Check sheet for the modelled part. Datum: model origin and axes. Units: mm. A direction names the side the tool comes from. Round coordinates to 2 decimals unless told otherwise and drop trailing zeros. Loops run counter-clockwise (first coordinate to the right, second up) from the corner with the lowest first, then second, coordinate; pieces in that order, holes last. Notation, with made-up numbers: (2, 50.25) - (49, 50.25) arc R15 cw to (49, 69.25) - close; hole circle Ø4 at (-11, -31). An arc over 180 degrees is marked (long way). Put each result on its own line as item: value.
```python
from build123d import *

# Parameters (mm, degrees)
SKETCH_1_W           = 1100
SKETCH_1_H           = 800
EXTRUDE_1_DEPTH      = 6
SKETCH_3_W           = 1100
SKETCH_3_H           = 800
SKETCH_3_W_2         = 1088
SKETCH_3_H_2         = 788
EXTRUDE_2_DEPTH      = 1200
SKETCH_4_W           = 900
SKETCH_4_H           = 800
EXTRUDE_3_DEPTH      = 4
SKETCH_5_W           = 50
SKETCH_5_H           = 50
EXTRUDE_4_DEPTH      = 950
EXTRUDE_5_DEPTH      = 19
EXTRUDE_5_DEPTH_BACK = 800
SKETCH_6_R           = 44.5
SKETCH_6_R_2         = 41
SKETCH_7_R           = 28.5
SKETCH_7_R_2         = 25
EXTRUDE_6_DEPTH      = 50
EXTRUDE_7_DEPTH      = 50
EXTRUDE_7_DEPTH_BACK = 50
SKETCH_8_R           = 16.75
SKETCH_8_R_2         = 13.55
SKETCH_9_R           = 21.15
SKETCH_9_R_2         = 17.95
EXTRUDE_8_DEPTH      = 49
SKETCH_10_R          = 16.75
SKETCH_10_R_2        = 13.55
EXTRUDE_9_DEPTH      = 30
SKETCH_13_W          = 1100
SKETCH_13_H          = 4
EXTRUDE_12_DEPTH     = 160
SKETCH_14_R          = 16.75
SKETCH_14_R_2        = 13.55
EXTRUDE_13_DEPTH     = 30


with BuildPart() as part:
    # Эскиз1 → Бобышка-Вытянуть1 (new body)
    with BuildSketch(Plane(origin=(0, 0, 0), x_dir=(1, 0, 0), z_dir=(0, 1, 0))):
        with Locations((550, 400)):
            Rectangle(SKETCH_1_W, SKETCH_1_H)
    extrude(amount=EXTRUDE_1_DEPTH)

    # Эскиз3 → Бобышка-Вытянуть2 (add)
    with BuildSketch(Plane(origin=(0, 6, 0), x_dir=(1, 0, 0), z_dir=(0, 1, 0))):
        with Locations((550, 400)):
            Rectangle(SKETCH_3_W, SKETCH_3_H)
        with Locations((550, 400)):
            Rectangle(SKETCH_3_W_2, SKETCH_3_H_2, mode=Mode.SUBTRACT)
    extrude(amount=EXTRUDE_2_DEPTH)

    # Эскиз4 → Бобышка-Вытянуть3 (add)
    with BuildSketch(Plane(origin=(0, 1206, 0), x_dir=(1, 0, 0), z_dir=(0, 1, 0))):
        with Locations((650, 400)):
            Rectangle(SKETCH_4_W, SKETCH_4_H)
    extrude(amount=EXTRUDE_3_DEPTH)

    # Эскиз5 → Бобышка-Вытянуть4 (add)
    with BuildSketch(Plane.XZ):
        with Locations((1075, -25)):
            Rectangle(SKETCH_5_W, SKETCH_5_H)
        with Locations((25, -25)):
            Rectangle(SKETCH_5_W, SKETCH_5_H)
        with Locations((1075, -775)):
            Rectangle(SKETCH_5_W, SKETCH_5_H)
        with Locations((25, -775)):
            Rectangle(SKETCH_5_W, SKETCH_5_H)
    extrude(amount=EXTRUDE_4_DEPTH)

    # Эскиз6 → Бобышка-Вытянуть5 (add, two sides: drawn at the far end of the back side and taken through both)
    with BuildSketch(Plane(origin=(0, 1210, 0), x_dir=(1, 0, 0), z_dir=(0, 1, 0)).offset(-EXTRUDE_5_DEPTH_BACK)):
        with Locations(Location((1000, 100, 0), (0, 0, 270))):
            Circle(SKETCH_6_R)
        with Locations(Location((1000, 100, 0), (0, 0, 270))):
            Circle(SKETCH_6_R_2, mode=Mode.SUBTRACT)
    extrude(amount=EXTRUDE_5_DEPTH + EXTRUDE_5_DEPTH_BACK)

    # Эскиз7 → Бобышка-Вытянуть6 (add)
    with BuildSketch(Plane.ZY):
        with Locations(Location((-250, 1160, 0), (0, 0, 180))):
            Circle(SKETCH_7_R)
        with Locations((-250, 1160)):
            Circle(SKETCH_7_R_2, mode=Mode.SUBTRACT)
    extrude(amount=EXTRUDE_6_DEPTH)

    # Эскиз8 → Бобышка-Вытянуть7 (add, two sides: drawn at the far end of the back side and taken through both)
    with BuildSketch(Plane.XZ.offset(-EXTRUDE_7_DEPTH_BACK)):
        with Locations(Location((171.2, -100, 0), (0, 0, 270))):
            Circle(SKETCH_8_R)
        with Locations(Location((171.2, -100, 0), (0, 0, 270))):
            Circle(SKETCH_8_R_2, mode=Mode.SUBTRACT)
    extrude(amount=EXTRUDE_7_DEPTH + EXTRUDE_7_DEPTH_BACK)

    # Эскиз9 → Бобышка-Вытянуть8 (add)
    with BuildSketch(Plane.XZ):
        with Locations(Location((300, -250, 0), (0, 0, 270))):
            Circle(SKETCH_9_R)
        with Locations(Location((300, -250, 0), (0, 0, 270))):
            Circle(SKETCH_9_R_2, mode=Mode.SUBTRACT)
    extrude(amount=EXTRUDE_8_DEPTH)

    # Эскиз10 → Бобышка-Вытянуть9 (add)
    with BuildSketch(Plane.XY):
        with Locations(Location((500, 1150, 0), (0, 0, 180))):
            Circle(SKETCH_10_R)
        with Locations((500, 1150)):
            Circle(SKETCH_10_R_2, mode=Mode.SUBTRACT)
    extrude(amount=EXTRUDE_9_DEPTH)

    # Эскиз13 → Бобышка-Вытянуть12 (add)
    with BuildSketch(Plane.XY):
        with Locations((550, -752)):
            Rectangle(SKETCH_13_W, SKETCH_13_H)
    extrude(amount=EXTRUDE_12_DEPTH)

    # Эскиз14 → Бобышка-Вытянуть13 (add)
    with BuildSketch(Plane.XY):
        with Locations(Location((550, 50, 0), (0, 0, 180))):
            Circle(SKETCH_14_R)
        with Locations((550, 50)):
            Circle(SKETCH_14_R_2, mode=Mode.SUBTRACT)
    extrude(amount=EXTRUDE_13_DEPTH)


solid = part.part
```
Item 1: Section check A-A on y = 583. Enter the section's corners in (x, z), then the cut area to 3 significant figures.
Filled sheet:
outline: (0, -800) - (1100, -800) - (1100, 0) - (0, 0) - close; circle Ø89 at (1000, -100); hole (6, -794) - (1094, -794) - (1094, -6) - (6, -6) - close; hole circle Ø82 at (1000, -100)
area: 23,600 mm²
Item 2: Section check C-C on z = -502.5. Enter the section's corners in (x, y).
Filled sheet:
outline: (0, 0) - (1100, 0) - (1100, 1210) - (200, 1210) - (200, 1206) - (1094, 1206) - (1094, 6) - (6, 6) - (6, 1206) - (0, 1206) - close
Item 3: Thickness scan on line 1 (Z direction, x = 171.2, y = 16); line 2 (Y direction, x = 550, z = 7.75); line 3 (Y direction, x = 687.5, z = -36). Record the ranges inside material, lowest first. Write a range as from..to.
Filled sheet:
line 1: -800..-794, -116.75..-113.55, -86.45..-83.25, -6..0
line 2: -754..-750, 33.25..36.45, 63.55..66.75
line 3: 0..6, 1206..1210
Item 4: Go/stop test with flat-tipped pins: pin 1 (10 mm diameter, centred on y = 33, z = -613.5, fed in from -X); pin 2 (8 mm diameter, centred on x = 521, z = -405.5, fed in from -Y). Record where each tip stops, or that it passes through.
Filled sheet:
pin 1: x = 0
pin 2: y = 0
Item 5: Tool access check on faces 1 (the cylindrical face through (956.56, 1219.37, -109.65)), 2 (the flat face through (25, -468, -50)), 3 (the flat face through (542, 6, -406)). Record the directions out of +Z, -Z, +X, -X, +Y, -Y that give a thin tool (end or side, any length) a straight path to the whole face; none if there is none.
Filled sheet:
face 1: +Y
face 2: +X, -X, -Y
face 3: none
Item 6: Release check for a two-part mould opening along Y. For faces 4 (the flat face through (3, 1206, -402)), 5 (the flat face through (641, 1206, -406)), 6 (the cylindrical face through (291.899, -24.157, -269.537)) record: +Y half, -Y half, draft (parallel to the pull), parting line (faces both ways), or undercut.
Filled sheet:
face 4: +Y half
face 5: undercut
face 6: draft
Item 7: Section check B-B on x = 906.5. Enter the section's corners in (y, z), then the cut area to 3 significant figures.
Filled sheet:
outline: (-754, 0) - (-750, 0) - (-750, 160) - (-754, 160) - close; (0, -800) - (1210, -800) - (1210, 0) - (0, 0) - close; hole (6, -794) - (1206, -794) - (1206, -6) - (6, -6) - close
area: 23,000 mm²
